Source: CAD feature listing. Evaluate the final solid. Frame: model axes, mm. Give positions to 0.01 mm unless a question says otherwise; leave off trailing zeros. Loops run counter-clockwise (first coordinate to the right, second up) from the corner with the lowest first, then second, coordinate; pieces in that order, holes last. Notation, with made-up numbers: M 8,-11.75 L 16,-11.75 A36 cw 16,23.25 Z; hole C 15.25,14.25 d10. An arc over 180 degrees is marked long. Put each result on its own line as item: value.
from build123d import *

# Parameters (mm, degrees)
SKETCH1_R           = 14
SKETCH1_R_2         = 1.025
SKETCH1_R_3         = 5
BOSS_EXTRUDE1_DEPTH = 1.22


with BuildPart() as part:
    # Sketch1 → Boss-Extrude1 (new body)
    with BuildSketch(Plane(origin=(0, 1.72, 0), x_dir=(1, 0, 0), z_dir=(0, 1, 0))):
        Circle(SKETCH1_R)
        with Locations((-8, 0)):
            Circle(SKETCH1_R_2, mode=Mode.SUBTRACT)
        with Locations((8, 0)):
            Circle(SKETCH1_R_2, mode=Mode.SUBTRACT)
        with Locations((-7.778174593, 7.778174593)):
            Circle(SKETCH1_R_2, mode=Mode.SUBTRACT)
        with Locations((-7.778174593, -7.778174593)):
            Circle(SKETCH1_R_2, mode=Mode.SUBTRACT)
        with Locations((7.778174593, -7.778174593)):
            Circle(SKETCH1_R_2, mode=Mode.SUBTRACT)
        with Locations((7.778174593, 7.778174593)):
            Circle(SKETCH1_R_2, mode=Mode.SUBTRACT)
        with Locations((0, 11)):
            Circle(SKETCH1_R_2, mode=Mode.SUBTRACT)
        with Locations((11, 0)):
            Circle(SKETCH1_R_2, mode=Mode.SUBTRACT)
        with Locations((0, -11)):
            Circle(SKETCH1_R_2, mode=Mode.SUBTRACT)
        with Locations((-11, 0)):
            Circle(SKETCH1_R_2, mode=Mode.SUBTRACT)
        with Locations((0, 8)):
            Circle(SKETCH1_R_2, mode=Mode.SUBTRACT)
        with Locations((0, -8)):
            Circle(SKETCH1_R_2, mode=Mode.SUBTRACT)
        Circle(SKETCH1_R_3, mode=Mode.SUBTRACT)
    extrude(amount=-BOSS_EXTRUDE1_DEPTH)


solid = part.part
1. Section query D-D (x = 11). Output: boundary loops of the cut face in (y, z) (3 decimals).
Found:
outline: M 0.5,-8.66 L 1.72,-8.66 L 1.72,-1.025 L 0.5,-1.025 Z; M 0.5,1.025 L 1.72,1.025 L 1.72,8.66 L 0.5,8.66 Z
2. Section query B-B (x = -8). Output: boundary loops of the cut face in (y, z) (3 decimals).
Found:
outline: M 0.5,-11.489 L 1.72,-11.489 L 1.72,-8.779 L 0.5,-8.779 Z; M 0.5,-6.777 L 1.72,-6.777 L 1.72,-1.025 L 0.5,-1.025 Z; M 0.5,1.025 L 1.72,1.025 L 1.72,6.777 L 0.5,6.777 Z; M 0.5,8.779 L 1.72,8.779 L 1.72,11.489 L 0.5,11.489 Z
3. Section query C-C (y = 0.9). State how many separate pieces and enclosed holes the cut face has, plus the area to 3 significant figures.
Found:
separate pieces: 1
enclosed holes: 13
area: 498 mm^2
4. Material intervals for line 1 (Z direction, x = 0, y = 1.1) (3 decimals); line 2 (X direction, y = 1.4, z = 8) (3 decimals), sorted ascending. Write a range as from..to.
Found:
line 1: -14..-12.025, -9.975..-9.025, -6.975..-5, 5..6.975, 9.025..9.975, 12.025..14
line 2: -11.489..-8.779, -6.777..-1.025, 1.025..6.777, 8.779..11.489
5. Contact query for a flat-ended pin moving along its axis: P1, Ø1.2, axis at x = 7.78, z = 7.78, coming from the +Y side. Output: stop coordinate, or through.
Found:
P1: through
6. Section query A-A (z = 0). Output: boundary loops of the cut face in (x, y) (3 decimals), plus the area to 3 significant figures.
Found:
outline: M -14,0.5 L -12.025,0.5 L -12.025,1.72 L -14,1.72 Z; M -9.975,0.5 L -9.025,0.5 L -9.025,1.72 L -9.975,1.72 Z; M -6.975,0.5 L -5,0.5 L -5,1.72 L -6.975,1.72 Z; M 5,0.5 L 6.975,0.5 L 6.975,1.72 L 5,1.72 Z; M 9.025,0.5 L 9.975,0.5 L 9.975,1.72 L 9.025,1.72 Z; M 12.025,0.5 L 14,0.5 L 14,1.72 L 12.025,1.72 Z
area: 12.0 mm^2
7. Draft query along Z for faces 1 (the cylindrical face through (-0.76, 1.12, 10.31)), 2 (the flat face through (0, 0.5, 6)), 3 (the cylindrical face through (12.932, 1.119, 5.362)). Return one class per face: pulls with the +Z half, pulls with the -Z half, needs draft (parallel to the pull), parting line crosses it, or undercut.
Found:
face 1: undercut
face 2: needs draft
face 3: parting line crosses it
